The listing builds one solid part. Answer for the finished solid, in the listing's coordinates (mm). A direction names the side the tool comes from. Give positions to 0.01 mm unless a question says otherwise; leave off trailing zeros. Loops run counter-clockwise (first coordinate to the right, second up) from the corner with the lowest first, then second, coordinate; pieces in that order, holes last. Notation, with made-up numbers: (-34, -14.5) - (-20, -14.5) arc R10 cw to (-20, -2.5) - close; hole circle Ø5 at (45.5, -40). An arc over 180 degrees is marked (long way). Answer as CSV lines item,"result". Start each with the question number.
1) Find the intervals of material crossed by line 1 along Z through (x, y) = (1.6, 35.5); line 2 along Z through (x, y) = (1.9, 37.5); line 3 along Z through (x, y) = (2.55, 58), in increasing order.
2) A cutting plane is placed at B-B (y = 8). Determine the outline of the cut face in (x, z), and give its area (3 significant figures).
3) A cutting plane is placed at D-D (y = 50). Determine the outline of the cut face in (x, z).
4) For faces 5 (the face through (2.465, 2.683, 20.531)), 6 (the face through (2.46, 35.25, 7.2)), 7 (the face through (2.46, 10.22, 33.5)), 8 (the face through (2.465, 34.704, 64.951)), 9 (the face through (2, 35, 0)), determine the directions among +Z, -Z, +X, -X, +Y, -Y from which every point of the face is accessible in a straight line to the end or side of a thin tool.
5) Flat-ended cylindrical pins translate along their axes: pin 1 (1.5 mm diameter, centred on x = 2.5, z = 35.5, fed in from +Y); pin 2 (1 mm diameter, centred on x = 4, y = 46, fed in from +Z); pin 3 (2 mm diameter, centred on x = 2.5, z = 59, fed in from -Y). Find the tip coordinate at first contact, or state that the pin passes through.
6) A cutting plane is placed at A-A (x = 2.45). Determine the outline of the cut face in (y, z).
7) For a pull along Y with two mould halves and no side action, classify faces 1 (the face through (2.465, 5.204, 27.857)), 2 (the face through (5, 27, 28)), 3 (the face through (2.465, 33.797, 20.044)), 4 (the face through (2.46, 27.72, 63.81)) as pulls with the +Y half, pulls with the -Y half, needs draft (parallel to the pull), parting line crosses it, or undercut.
8) A cutting plane is placed at C-C (y = 58.5). Determine the outline of the cut face in (x, z), and give its area (3 significant figures).
```python
from build123d import *

# Parameters (mm, degrees)
F1_DEPTH = 5


with BuildPart() as f1:
    # F0 (on Right) → F1 (new body)
    with BuildSketch(Plane.YZ):
        with BuildLine():
            Line((4, 19.770527), (0, 12.842323))
            Line((0, 12.842323), (0, 0))
            Line((0, 0), (70, 0))
            Line((70, 0), (70, 3))
            ThreePointArc((70, 3), (69.12132, 5.12132), (67, 6))
            Line((67, 6), (38.500565, 6))
            ThreePointArc((38.500565, 6), (35.21584, 7.230308), (33.547604, 10.315768))
            ThreePointArc((33.547604, 10.315768), (33.8233, 20.180017), (37.28461, 29.421162))
            Line((37.28461, 29.421162), (52.28461, 55.401924))
            ThreePointArc((52.28461, 55.401924), (52.584311, 57.678381), (51.186533, 59.5))
            Line((51.186533, 59.5), (33, 70))
            Line((33, 70), (29, 63.071797))
            Line((29, 63.071797), (26.401924, 64.571797))
            Line((26.401924, 64.571797), (18.901924, 51.581416))
            Line((18.901924, 51.581416), (21.5, 50.081416))
            Line((21.5, 50.081416), (11.5, 32.760908))
            Line((11.5, 32.760908), (8.901924, 34.260908))
            Line((8.901924, 34.260908), (1.401924, 21.270527))
            Line((1.401924, 21.270527), (4, 19.770527))
        make_face()
        Polygon((4.464102, 12.574374), (5.964102, 15.17245), (14.624356, 10.17245), (13.124356, 7.574374), align=None, mode=Mode.SUBTRACT)
        Polygon((33.964102, 63.669873), (35.464102, 66.267949), (44.124356, 61.267949), (42.624356, 58.669873), align=None, mode=Mode.SUBTRACT)
    extrude(amount=F1_DEPTH)


solid = f1.part
```
Ans:
1,line 1,"0 to 7, 25.78 to 62.78, 66.25 to 68.56"
1,line 2,"0 to 6.1, 29.79 to 61.63, 65.09 to 67.4"
1,line 3,"0 to 6"
2,outline,"(0, 0) - (5, 0) - (5, 10.53) - (0, 10.53) - close; (0, 14) - (5, 14) - (5, 32.7) - (0, 32.7) - close"
2,area,"146 mm2"
3,outline,"(0, 0) - (5, 0) - (5, 6) - (0, 6) - close; (0, 51.44) - (5, 51.44) - (5, 60.19) - (0, 60.19) - close"
4,face 5,"+X, -X, -Y"
4,face 6,"+X, -X, +Y"
4,face 7,"+Z, +X, -X"
4,face 8,"+X, -X"
4,face 9,"-Z, +X, -X, +Y, -Y"
5,pin 1,"y = 41.23"
5,pin 2,"z = 62.78"
5,pin 3,"y = 22.61"
6,outline,"(0, 0) - (70, 0) - (70, 3) arc R3 ccw to (67, 6) - (38.5, 6) arc R5 cw to (33.55, 10.32) arc R30 cw to (37.28, 29.42) - (52.28, 55.4) arc R3 ccw to (51.19, 59.5) - (33, 70) - (29, 63.07) - (26.4, 64.57) - (18.9, 51.58) - (21.5, 50.08) - (11.5, 32.76) - (8.9, 34.26) - (1.4, 21.27) - (4, 19.77) - (0, 12.84) - close; hole (4.46, 12.57) - (13.12, 7.57) - (14.62, 10.17) - (5.96, 15.17) - close; hole (33.96, 63.67) - (42.62, 58.67) - (44.12, 61.27) - (35.46, 66.27) - close"
7,face 1,"pulls with the -Y half"
7,face 2,"needs draft"
7,face 3,"pulls with the +Y half"
7,face 4,"undercut"
8,outline,"(0, 0) - (5, 0) - (5, 6) - (0, 6) - close"
8,area,"30.0 mm2"
